Work out the finished part from the listing and answer in its coordinate system (mm). Coordinates: 2 decimals unless noted, no trailing zeros. Loops run counter-clockwise (first coordinate to the right, second up) from the corner with the lowest first, then second, coordinate; pieces in that order, holes last. Notation, with made-up numbers: (9, 69.25) -> (48, 69.25) arc R28 cw to (48, 107.25) -> close; hole circle Ø11 at (78.25, -18). An arc over 180 degrees is marked (long way). Use a Markdown table: item, result.
from build123d import *

# Parameters (mm, degrees)
SKETCH1_W           = 4.5
SKETCH1_H           = 7
BOSS_EXTRUDE1_DEPTH = 2
SKETCH2_W           = 1.5
SKETCH2_H           = 7
CUT_EXTRUDE3_DEPTH  = 0.5
CUT_EXTRUDE4_DEPTH  = 9.250795932


with BuildPart() as part:
    # Sketch1 → Boss-Extrude1 (new body)
    with BuildSketch(Plane(origin=(0, 0, 0), x_dir=(1, 0, 0), z_dir=(0, 1, 0))):
        with Locations((1.632735313, 5.351794061)):
            Rectangle(SKETCH1_W, SKETCH1_H)
    extrude(amount=BOSS_EXTRUDE1_DEPTH)

    # Sketch2 → Cut-Extrude3 (cut)
    with BuildSketch(Plane(origin=(0, 2, 0), x_dir=(1, 0, 0), z_dir=(0, 1, 0))):
        with Locations((1.632735313, 5.351794061)):
            Rectangle(SKETCH2_W, SKETCH2_H)
    extrude(amount=-CUT_EXTRUDE3_DEPTH, mode=Mode.SUBTRACT)

    # Sketch3 → Cut-Extrude4 (cut, through all)
    with BuildSketch(Plane(origin=(0, 0, -8.851794061), x_dir=(-1, 0, 0), z_dir=(0, 0, -1))):
        Polygon((0.617264687, 2), (-0.132735313, 0.700961894), (0.617264687, 0.700961894), align=None)
        Polygon((-3.882735313, 2), (-3.132735313, 0.700961894), (-3.882735313, 0.700961894), align=None)
    extrude(amount=-CUT_EXTRUDE4_DEPTH, mode=Mode.SUBTRACT)


solid = part.part
Q1. Determine the mould class of faces 1 (the flat face through (-0.25, 1.36, -5.4)), 2 (the flat face through (2, 1.5, -5)), 3 (the flat face through (3.513, 1.36, -5.401)), 4 (the flat face through (2, 1, -8.852)) for opening direction X: pulls with the +X half, pulls with the -X half, needs draft (parallel to the pull), parting line crosses it, or undercut.
Solved:
| item | result |
|---|---|
| face 1 | pulls with the -X half |
| face 2 | undercut |
| face 3 | pulls with the +X half |
| face 4 | needs draft |
Q2. Section B-B on y = 1.6 is taken. Determine the outline of the cut face in (x, z), and give its area (3 significant figures).
Solved:
| item | result |
|---|---|
| outline | (-0.39, -8.85) -> (0.88, -8.85) -> (0.88, -1.85) -> (-0.39, -1.85) -> close; (2.38, -8.85) -> (3.65, -8.85) -> (3.65, -1.85) -> (2.38, -1.85) -> close |
| area | 17.8 mm² |
Q3. Section A-A on x = 3.5 is taken. Determine the outline of the cut face in (y, z), and give its area (3 significant figures).
Solved:
| item | result |
|---|---|
| outline | (0, -8.85) -> (0.7, -8.85) -> (0.7, -1.85) -> (0, -1.85) -> close; (1.34, -8.85) -> (2, -8.85) -> (2, -1.85) -> (1.34, -1.85) -> close |
| area | 9.55 mm² |
Q4. Section D-D on x = 1.65 is taken. Determine the outline of the cut face in (y, z), and give its area (3 significant figures).
Solved:
| item | result |
|---|---|
| outline | (0, -8.85) -> (1.5, -8.85) -> (1.5, -1.85) -> (0, -1.85) -> close |
| area | 10.5 mm² |
Q5. Consider line 1 (Y direction, x = 1.35, z = -5); line 2 (X direction, y = 1.85, z = -7); line 3 (Y direction, x = -0.25, z = -6.5). Determine where each line is inside the solid, lowest interval first. Write a range as [from, to].
Solved:
| item | result |
|---|---|
| line 1 | [0, 1.5] |
| line 2 | [-0.53, 0.88], [2.38, 3.8] |
| line 3 | [0, 0.7], [1.36, 2] |
Q6. Section C-C on z = -8 is taken. Determine the outline of the cut face in (x, y).
Solved:
| item | result |
|---|---|
| outline | (-0.62, 0) -> (3.88, 0) -> (3.88, 0.7) -> (3.13, 0.7) -> (3.88, 2) -> (2.38, 2) -> (2.38, 1.5) -> (0.88, 1.5) -> (0.88, 2) -> (-0.62, 2) -> (0.13, 0.7) -> (-0.62, 0.7) -> close |
